The drawing under review shows one solid part. Ordinate dimensions are in mm from its lowest x, y, z. A direction names the side the tool comes from. Round coordinates to 2 decimals unless told otherwise and drop trailing zeros. Order: outer loops, then holes, each group sorted by start corner. A loop starts at its lowest first (then second) coordinate and runs counter-clockwise, first axis right, second up. Notation, with made-up numbers: M -35.75,10 L -29.75,10 A20 ccw -29.75,42 Z; hole C -27,-1 d6. An arc over 180 degrees is marked long. Answer as a JSON object with one key per item and string values. Group by question number.
1. Add section B-B on y = 5.55. State the section outline as (x, z) points, and give its area (3 significant figures).
2. Add section D-D on y = 3. State the section outline as (x, z) points, and give its area (3 significant figures).
3. Add section A-A on x = 26.5. State the section outline as (y, z) points.
4. Machinability: for the marked faces 1, 2 and 3, which of the approach directions +Z, -Z, +X, -X, +Y, -Y give a long, thin tool a straight path to every point of the face, cutting with its end or side? Answer none if there is none.
5. Clearance check with flat-ended pins moving along their axes: P1, Ø1.8, axis at x = 39, y = 4, coming from the +Z side; P2, Ø1, axis at x = 22, y = 5, coming from the -Z side; P3, Ø8, axis at x = 11.5, z = 17.5, coming from the +Y side; P4, Ø1, axis at y = 2.5, z = 26.5, coming from the +X side. State where each tip first meets the part, or that it passes through.
6. Mouldability with a two-part tool opening along X and no side actions: class the marked faces 4, 5, 6 and 7 as released by +X, released by -X, zero draft, split by the parting line, or undercut.
7. Add section C-C on z = 15.5. State the section outline as (x, y) points, and give its area (3 significant figures).
8. To check wall thickness, follow probe 1 along X at (y, z) = (0.75, 16); probe 2 along Y at (x, z) = (23, 28.5); probe 3 along Z at (x, y) = (40.5, 1.45). State the ranges of each line that lie inside material, in increasing order. Write a range as [from, to].
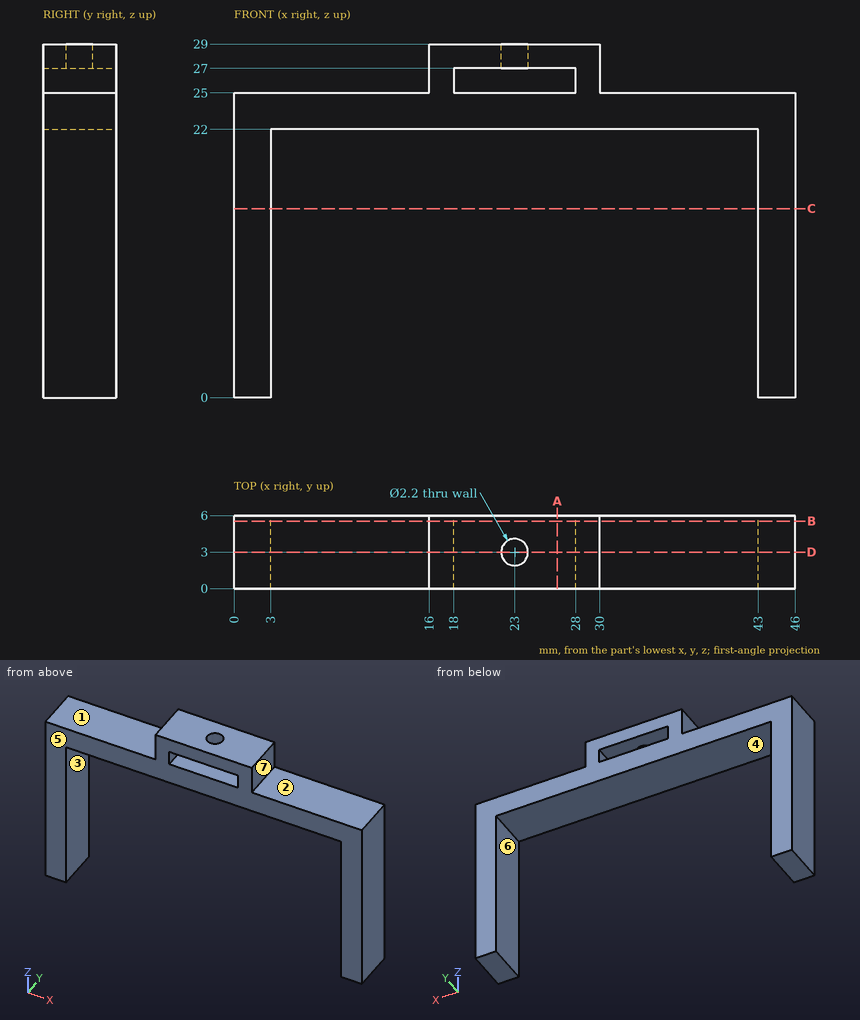
Recorded:
{
 "1": {"outline": "M 0,0 L 3,0 L 3,22 L 43,22 L 43,0 L 46,0 L 46,25 L 30,25 L 30,29 L 16,29 L 16,25 L 0,25 Z; hole M 18,25 L 28,25 L 28,27 L 18,27 Z", "area": "306 mm²"},
 "2": {"outline": "M 0,0 L 3,0 L 3,22 L 43,22 L 43,0 L 46,0 L 46,25 L 30,25 L 30,29 L 24.1,29 L 24.1,27 L 28,27 L 28,25 L 18,25 L 18,27 L 21.9,27 L 21.9,29 L 16,29 L 16,25 L 0,25 Z", "area": "302 mm²"},
 "3": {"outline": "M 0,22 L 6,22 L 6,25 L 0,25 Z; M 0,27 L 6,27 L 6,29 L 0,29 Z"},
 "4": {"face 1": "+Z, -X, +Y, -Y", "face 2": "+Z, +X, +Y, -Y", "face 3": "-Z, +Y, -Y"},
 "5": {"P1": "stops at z = 25", "P2": "stops at z = 22", "P3": "passes through", "P4": "stops at x = 30"},
 "6": {"face 4": "undercut", "face 5": "zero draft", "face 6": "undercut", "face 7": "released by +X"},
 "7": {"outline": "M 0,0 L 3,0 L 3,6 L 0,6 Z; M 43,0 L 46,0 L 46,6 L 43,6 Z", "area": "36.0 mm²"},
 "8": {"probe 1": "x = [0, 3], [43, 46]", "probe 2": "y = [0, 1.9], [4.1, 6]", "probe 3": "z = [22, 25]"}
}
